The model under review builds one solid part; all positions refer to its coordinate system, in mm. Face numbers are marked on the shaded views. A direction names the side the tool comes from. Coordinates: 2 decimals unless noted, no trailing zeros. Write each loop counter-clockwise with the first axis right and the second up, starting at its lowest first coordinate (ties: lowest second). Pieces come first, ordered by that corner, then holes.
1) For line 1 (Y direction, x = 14, z = 0.6); line 2 (Z direction, x = -5.5, y = -3); line 3 (Y direction, x = -10, z = 3.1), list the stretches that pass through material, from the lowest coordinate up.
2) Add section B-B, the plane x = -14. State the section outline as (y, z) points, then the cut area to 3 significant figures.
3) Add section D-D, the plane z = 21.5. State the section outline as (x, y) points, then the cut area to 3 significant figures.
4) Add section A-A, the plane y = 14. State the section outline as (x, z) points, then the cut area to 4 significant figures.
5) Machinability: for the marked faces 1, 2 and 3, which of the approach directions +Z, -Z, +X, -X, +Y, -Y give a long, thin tool a straight path to every point of the face, cutting with its end or side? Answer none if there is none.
6) For P1, Ø12, axis at y = 0.5, z = 13.5, coming from the -X side; P2, Ø2, axis at x = 14, y = 14, coming from the -Z side; P3, Ø0.6, axis at x = -8.5, z = 3.5, coming from the +Y side; P4, Ø8, axis at y = -4, z = 11, coming from the +X side, all flat-tipped, find the tip position at first contact; note any pin that passes through.
7) Add section C-C, the plane z = 1. State the section outline as (x, y) points.
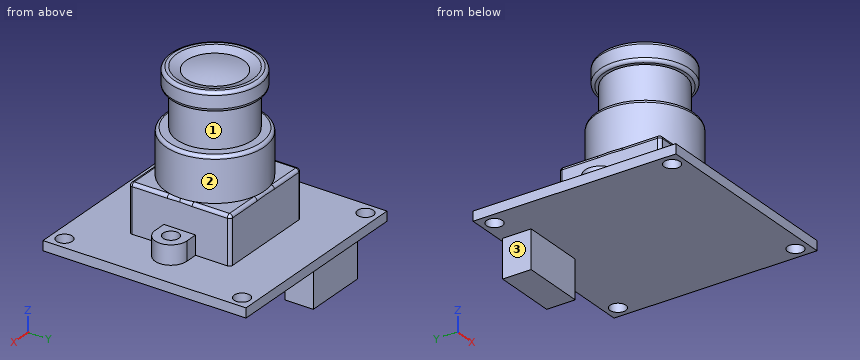
from build123d import *

# Parameters (mm, degrees)
SKETCH1_W           = 32
SKETCH1_H           = 32
BOSS_EXTRUDE1_DEPTH = 1.5
SKETCH2_R           = 1.25
CUT_EXTRUDE1_DEPTH  = 2.5
SKETCH3_W           = 16
SKETCH3_H           = 16
BOSS_EXTRUDE2_DEPTH = 7.5
SKETCH4_R           = 1.25
BOSS_EXTRUDE3_DEPTH = 3
SKETCH5_R           = 7.75
BOSS_EXTRUDE4_DEPTH = 7
SKETCH6_R           = 6
BOSS_EXTRUDE5_DEPTH = 6
SKETCH9_W           = 10
SKETCH9_H           = 4.5
BOSS_EXTRUDE6_DEPTH = 6
FILLET1_R           = 0.5
FILLET2_R           = 0.5


with BuildPart() as part:
    # Sketch1 → Boss-Extrude1 (new body)
    with BuildSketch(Plane.XY):
        Rectangle(SKETCH1_W, SKETCH1_H)
    extrude(amount=BOSS_EXTRUDE1_DEPTH)

    # Sketch2 → Cut-Extrude1 (cut, through all)
    with BuildSketch(Plane.XY.offset(1.5)):
        with Locations((-14, 14)):
            Circle(SKETCH2_R)
        with Locations((14, 14)):
            Circle(SKETCH2_R)
        with Locations((14, -14)):
            Circle(SKETCH2_R)
        with Locations((-14, -14)):
            Circle(SKETCH2_R)
    extrude(amount=-CUT_EXTRUDE1_DEPTH, mode=Mode.SUBTRACT)

    # Sketch3 → Boss-Extrude2 (add)
    with BuildSketch(Plane.XY.offset(1.5)):
        Rectangle(SKETCH3_W, SKETCH3_H)
    extrude(amount=BOSS_EXTRUDE2_DEPTH)

    # Sketch4 → Boss-Extrude3 (add)
    with BuildSketch(Plane.XY.offset(1.5)):
        with BuildLine():
            Line((-10, 2.5), (-8, 2.5))
            Line((-8, 2.5), (-8, -2.5))
            Line((-8, -2.5), (-10, -2.5))
            ThreePointArc((-10, -2.5), (-12.5, 0), (-10, 2.5))
        make_face()
        with Locations((-10, 0)):
            Circle(SKETCH4_R, mode=Mode.SUBTRACT)
        with BuildLine():
            Line((10, -2.5), (8, -2.5))
            Line((8, -2.5), (8, 2.5))
            Line((8, 2.5), (10, 2.5))
            ThreePointArc((10, 2.5), (12.5, 0), (10, -2.5))
        make_face()
        with Locations((10, 0)):
            Circle(SKETCH4_R, mode=Mode.SUBTRACT)
    extrude(amount=BOSS_EXTRUDE3_DEPTH)

    # Sketch5 → Boss-Extrude4 (add)
    with BuildSketch(Plane.XY.offset(9)):
        Circle(SKETCH5_R)
    extrude(amount=BOSS_EXTRUDE4_DEPTH)

    # Sketch6 → Boss-Extrude5 (add)
    with BuildSketch(Plane.XY.offset(16)):
        Circle(SKETCH6_R)
    extrude(amount=BOSS_EXTRUDE5_DEPTH)

    # Sketch8 → Revolve1 (revolve)
    with BuildSketch(Plane(origin=(0, 0, 0), x_dir=(1, 0, 0), z_dir=(0, 1, 0))):
        with BuildLine():
            ThreePointArc((0, -25), (-2.263846285, -24.874616561), (-4.5, -24.5))
            Line((-4.5, -24.5), (-6, -25))
            Line((-6, -25), (-7, -25))
            Line((-7, -25), (-7, -22))
            Line((-7, -22), (0, -22))
            Line((0, -22), (0, -25))
        make_face()
    revolve(axis=Axis((0, 0, 22), (0, 0, 1)))

    # Sketch9 → Boss-Extrude6 (add)
    with BuildSketch(Plane(origin=(0, 0, 0), x_dir=(-1, 0, 0), z_dir=(0, 0, -1))):
        with Locations((5, 13.25)):
            Rectangle(SKETCH9_W, SKETCH9_H)
    extrude(amount=BOSS_EXTRUDE6_DEPTH)

    # Fillet1
    fillet1_edges = [part.edges().sort_by_distance(p)[0] for p in [
        (-8, 8, 5.25),
        (-8, -8, 5.25),
        (8, -8, 5.25),
        (8, 8, 5.25),
    ]]
    fillet(fillet1_edges, radius=FILLET1_R)

    # Fillet2
    fillet2_edges = [part.edges().sort_by_distance(p)[0] for p in [
        (0, -8, 9),
        (-8, 0, 9),
        (8, 0, 9),
        (0, 8, 9),
        (7.853553391, 7.853553391, 9),
        (7.853553391, -7.853553391, 9),
        (-7.853553391, 7.853553391, 9),
        (-7.853553391, -7.853553391, 9),
        (-7.75, 0, 16),
        (7, 0, 22),
        (7, 0, 25),
    ]]
    fillet(fillet2_edges, radius=FILLET2_R)


solid = part.part
Geometry results:
1. line 1: y = -16 to -15.25, -12.75 to 12.75, 15.25 to 16
1. line 2: z = 0 to 16, 22 to 25
1. line 3: y = -2.5 to -1.25, 1.25 to 2.5
2. outline: (-16, 0) - (-15.25, 0) - (-15.25, 1.5) - (-16, 1.5) - close; (-12.75, 0) - (12.75, 0) - (12.75, 1.5) - (-12.75, 1.5) - close; (15.25, 0) - (16, 0) - (16, 1.5) - (15.25, 1.5) - close
2. area: 40.5 mm2
3. outline: circle Ø12 at (0, 0)
3. area: 113 mm2
4. outline: (-16, 0) - (-15.25, 0) - (-15.25, 1.5) - (-16, 1.5) - close; (-12.75, 0) - (-10, 0) - (-10, -6) - (0, -6) - (0, 0) - (12.75, 0) - (12.75, 1.5) - (-12.75, 1.5) - close; (15.25, 0) - (16, 0) - (16, 1.5) - (15.25, 1.5) - close
4. area: 100.5 mm2
5. face 1: none
5. face 2: +Z
5. face 3: -Z, -X, +Y, -Y
6. P1: stops at x = -8
6. P2: passes through
6. P3: stops at y = 2.5
6. P4: stops at x = 8
7. outline: (-16, -16) - (16, -16) - (16, 16) - (-16, 16) - close; hole circle Ø2.5 at (-14, -14); hole circle Ø2.5 at (-14, 14); hole circle Ø2.5 at (14, -14); hole circle Ø2.5 at (14, 14)
